Input: part model. Units: mm. Frame: model coordinates. Face numbers are marked on the shaded views. A direction names the side the tool comes from. Round coordinates to 2 decimals unless told otherwise and drop trailing zeros. Loops run counter-clockwise (first coordinate to the right, second up) from the corner with the lowest first, then second, coordinate; pieces in that order, holes last.
1) First-contact query: pin 1 (5.5 mm diameter, centred on x = -11.5, z = 23.5, fed in from +Y); pin 2 (8 mm diameter, centred on x = 11, z = 25, fed in from -Y); pin 3 (2 mm diameter, centred on x = -7.5, y = -15, fed in from +Z). Flat tips, straight axial feed; report the tip coordinate or a pass-through.
2) Draft query along Z for the marked faces 1, 2, 3 and 4. Return one class per face: pulls with the +Z half, pulls with the -Z half, needs draft (parallel to the pull), parting line crosses it, or undercut.
3) Section D-D, the plane x = 4. Return loops of the section in (y, z).
4) Section A-A, the plane z = 6. Return loops of the section in (x, y), and give its area (3 significant figures).
5) Access query for the marked faces 5, 6 and 7. Directions: +Z, -Z, +X, -X, +Y, -Y. A direction counts if a zero-diameter tool reaches every point of the face in a straight line with its end or side. Return the directions, or none.
6) Section B-B, the plane y = 0. Return loops of the section in (x, z).
7) Ray query, line 1 along Y through (x, z) = (0, 5); line 2 along Z through (x, y) = (4.75, -8); line 3 along Y through (x, z) = (-7.5, 46.25). Return the intervals inside material, ascending.
8) Section C-C, the plane z = 25. Return loops of the section in (x, y), and give its area (3 significant figures).
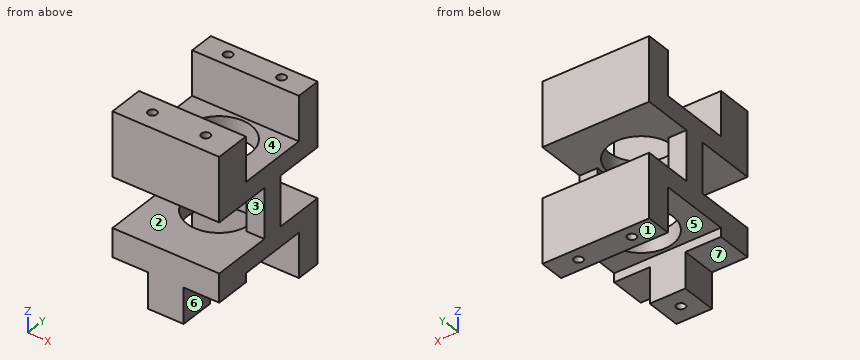
Autodesk Inventor part; units mm, degrees
ref_plane "YZ Plane" through (0, 0, 0) normal (1, 0, 0) x (0, 1, 0)
ref_plane "XZ Plane" through (0, 0, 0) normal (0, 1, 0) x (-1, 0, 0)
ref_plane "XY Plane" through (0, 0, 0) normal (0, 0, 1) x (1, 0, 0)
sketch "Sketch1" plane through (0, 0, 0) normal (0, 0, 1) x (1, 0, 0)
  line L0 (-15, 17) -> (15, 17)
  line L1 (15, 17) -> (15, -20)
  line L2 (15, -20) -> (-15, -20)
  line L3 (-15, -20) -> (-15, 17)
  point P0 (0, 0)
  dimension "d0" = 37
  dimension "d1" = 30
  dimension "d2" = 15
  dimension "d3" = 20
extrude "Extrusion1" add sketch "Sketch1" along normal blind 50
sketch "Sketch2" plane through (0, 0, 50) normal (0, 0, 1) x (1, 0, 0)
  circle A0 centre (0, 0) radius 9
  dimension "d6" = 18
extrude "Extrusion2" cut sketch "Sketch2" against normal through all
sketch "Sketch3" plane through (15, -20, 0) normal (1, 0, 0) x (0, 0, -1)
  line L0 (-50, 30) -> (-37.5, 30)
  line L1 (-37.5, 30) -> (-37.5, 10)
  line L2 (-37.5, 10) -> (-50, 10)
  line L3 (-50, 10) -> (-50, 30)
  line L4 (0, 0) -> (0, 37)
  line L5 (0, 30) -> (-12.5, 30)
  line L6 (-12.5, 30) -> (-12.5, 10)
  line L7 (-12.5, 10) -> (0, 10)
  line L8 (0, 10) -> (0, 30)
  line L9 (0, 0) -> (-50, 0)
  line L10 (0, 37) -> (-50, 37)
  line L11 (-50, 0) -> (-50, 37)
  point P0 (0, 20)
  dimension "d9" = 10
  dimension "d10" = 7
  dimension "d11" = 10
  dimension "d12" = 0
  dimension "d13" = 12.5
  dimension "d14" = 12.5
extrude "Extrusion3" cut sketch "Sketch3" against normal through all contours L0 L1 L2 L3 | L4 L7 L6 L5
sketch "Sketch4" plane through (15, -20, 50) normal (1, 0, 0) x (0, 0, -1)
  line L0 (18, 37) -> (32, 37)
  line L1 (32, 37) -> (32, 23)
  line L2 (32, 23) -> (18, 23)
  line L3 (18, 23) -> (18, 37)
  line L4 (18, 0) -> (32, 0)
  line L5 (32, 0) -> (32, 17)
  line L6 (32, 17) -> (18, 17)
  line L7 (18, 17) -> (18, 0)
  line L8 (50, 37) -> (0, 37)
  line L9 (50, 0) -> (0, 0)
  line L10 (0, 30) -> (0, 37)
  point P0 (50, 20)
  dimension "d17" = 14
  dimension "d18" = 0
  dimension "d19" = 0
  dimension "d20" = 18
  dimension "d21" = 17
  dimension "d22" = 14
extrude "Extrusion4" cut sketch "Sketch4" against normal through all
sketch "Sketch5" plane through (0, 0, 0) normal (0, 0, -1) x (-1, 0, 0)
  line L0 (-15, -20) -> (15, -20)
  line L1 (-15, -20) -> (-5, -20)
  line L2 (-5, -20) -> (-5, -10)
  line L3 (-5, -10) -> (-15, -10)
  line L4 (-15, -10) -> (-15, -20)
  line L5 (15, -20) -> (5, -20)
  line L6 (5, -20) -> (5, -10)
  line L7 (5, -10) -> (15, -10)
  line L8 (15, -10) -> (15, -20)
  line L9 (15, -10) -> (-15, -10)
  point P0 (0, 0)
  dimension "d27" = 10
  dimension "d28" = 10
  dimension "d31" = 0
  dimension "d32" = 0
extrude "Extrusion5" cut sketch "Sketch5" against normal blind 10 contours L4 L3 L2 L0 | L6 L7 L8 L0
sketch "Sketch6" plane through (0, 0, 50) normal (0, 0, 1) x (1, 0, 0)
  line L0 (15, 17) -> (-15, 17)
  line L1 (-15, 17) -> (-15, 10)
  line L2 (-15, -10) -> (-15, -20)
  line L3 (-15, -20) -> (15, -20)
  point P0 (0, 0)
  point P1 (-7.5, 13.5)
  point P2 (7.5, 13.5)
  point P3 (-7.5, -15)
  point P4 (7.5, -15)
  dimension "d33" = 3.5
  dimension "d34" = 3.5
  dimension "d35" = 15
  dimension "d36" = 7.5
  dimension "d37" = 7.5
  dimension "d38" = 15
  dimension "d39" = 5
  dimension "d40" = 5
hole "Hole1" at (-7.5, 13.5, 50) at (7.5, 13.5, 50) at (-7.5, -15, 50) at (7.5, -15, 50) direction (0, 0, -1) diameter 2.459 depth 8 tip angle 118
sketch "Sketch7" plane through (0, 0, 0) normal (0, 0, -1) x (-1, 0, 0)
  circle A0 centre (-7.5, 13.5) radius 1.2295
  circle A1 centre (7.5, 13.5) radius 1.2295
  point P0 (0, 0)
  point P1 (0, -15)
  dimension "d49" = 15
  dimension "d50" = 0
hole "Hole2" at (7.5, 13.5, 0) at (-7.5, 13.5, 0) at (0, -15, 0) direction (0, 0, 1) diameter 2.459 depth 8 tip angle 118
sketch "Sketch8" plane through (-15, 3, 18) normal (0, 1, 0) x (1, 0, 0)
  line L0 (30, -14) -> (23.4853, -14)
  line L1 (5, 0) -> (25, 0)
  line L2 (25, 0) -> (25, -14)
  line L3 (25, -14) -> (5, -14)
  line L4 (5, -14) -> (5, 0)
  line L5 (0, 0) -> (30, 0)
  line L6 (23.4853, -14) -> (23.4853, 0)
  line L7 (6.5147, 0) -> (6.5147, -14)
  line L8 (30, 0) -> (30, -14)
  line L9 (0, -14) -> (0, 0)
  point P0 (15, 18)
  dimension "d58" = 0
  dimension "d63" = 5
  dimension "d64" = 5
extrude "Extrusion6" cut sketch "Sketch8" against normal through all contours L0 L6 L1 L2 | L3 L4 L1 L7
properties part number "RotationShell"
Final values:
1. pin 1: stops at y = 3
1. pin 2: stops at y = -3
1. pin 3: stops at z = 41.86
2. face 1: pulls with the -Z half
2. face 2: undercut
2. face 3: undercut
2. face 4: pulls with the +Z half
3. outline: (-20, 0) - (-10, 0) - (-10, 12.5) - (-8.06, 12.5) - (-8.06, 18) - (-20, 18) - close; (-20, 32) - (-8.06, 32) - (-8.06, 37.5) - (-10, 37.5) - (-10, 50) - (-20, 50) - close; (8.06, 12.5) - (10, 12.5) - (10, 0) - (17, 0) - (17, 18) - (8.06, 18) - close; (8.06, 32) - (17, 32) - (17, 50) - (10, 50) - (10, 37.5) - (8.06, 37.5) - close
4. outline: (-15, 10) - (15, 10) - (15, 17) - (-15, 17) - close; (-5, -20) - (5, -20) - (5, -10) - (-5, -10) - close; hole circle Ø2.46 at (-7.5, 13.5); hole circle Ø2.46 at (0, -15); hole circle Ø2.46 at (7.5, 13.5)
4. area: 296 mm2
5. face 5: -Z, +X, -X
5. face 6: -Z, +X, -Y
5. face 7: -Z, -X, -Y
6. outline: (-15, 12.5) - (-9, 12.5) - (-9, 18) - (-10, 18) - (-10, 32) - (-9, 32) - (-9, 37.5) - (-15, 37.5) - close; (9, 12.5) - (15, 12.5) - (15, 37.5) - (9, 37.5) - (9, 32) - (10, 32) - (10, 18) - (9, 18) - close
7. line 1: y = -20 to -16.23, -13.77 to -10, 10 to 17
7. line 2: z = 12.5 to 18, 32 to 37.5
7. line 3: y = -20 to -16.23, -13.77 to -10, 10 to 12.27, 14.73 to 17
8. outline: (-15, -3) - (-10, -3) - (-10, 3) - (-15, 3) - close; (10, -3) - (15, -3) - (15, 3) - (10, 3) - close
8. area: 60.0 mm2
